from build123d import *

# Parameters (mm, degrees)
SKETCH1_R           = 2.5
BOSS_EXTRUDE1_DEPTH = 4
FILLET1_R           = 10.16


with BuildPart() as part:
    # Sketch1 → Boss-Extrude1 (new body)
    with BuildSketch(Plane(origin=(0, 25.4, 0), x_dir=(1, 0, 0), z_dir=(0, 1, 0))):
        Polygon((-190.5, -241.3), (-190.5, -279.4), (-190.5, -304.8), (-63.5, -304.8), (-63.5, -279.4), (-101.6, -279.4), (-101.6, -241.3), (-127, -241.3), (-127, -279.4), (-165.1, -279.4), (-165.1, -241.3), align=None)
        with Locations((-114.3, -292.1)):
            Circle(SKETCH1_R, mode=Mode.SUBTRACT)
        with Locations((-177.8, -292.1)):
            Circle(SKETCH1_R, mode=Mode.SUBTRACT)
        with Locations((-158.75, -292.1)):
            Circle(SKETCH1_R, mode=Mode.SUBTRACT)
        with Locations((-95.25, -292.1)):
            Circle(SKETCH1_R, mode=Mode.SUBTRACT)
        with Locations((-139.7, -292.1)):
            Circle(SKETCH1_R, mode=Mode.SUBTRACT)
        with Locations((-76.2, -292.1)):
            Circle(SKETCH1_R, mode=Mode.SUBTRACT)
        with Locations((-114.3, -273.05)):
            Circle(SKETCH1_R, mode=Mode.SUBTRACT)
        with Locations((-177.8, -273.05)):
            Circle(SKETCH1_R, mode=Mode.SUBTRACT)
        with Locations((-114.3, -254)):
            Circle(SKETCH1_R, mode=Mode.SUBTRACT)
        with Locations((-177.8, -254)):
            Circle(SKETCH1_R, mode=Mode.SUBTRACT)
    extrude(amount=BOSS_EXTRUDE1_DEPTH)

    # Fillet1
    fillet1_edges = [part.edges().sort_by_distance(p)[0] for p in [
        (-190.5, 27.4, 304.8),
        (-190.5, 27.4, 241.3),
        (-165.1, 27.4, 241.3),
        (-165.1, 27.4, 279.4),
        (-127, 27.4, 279.4),
        (-127, 27.4, 241.3),
        (-101.6, 27.4, 241.3),
        (-101.6, 27.4, 279.4),
        (-63.5, 27.4, 279.4),
        (-63.5, 27.4, 304.8),
    ]]
    fillet(fillet1_edges, radius=FILLET1_R)


solid = part.part
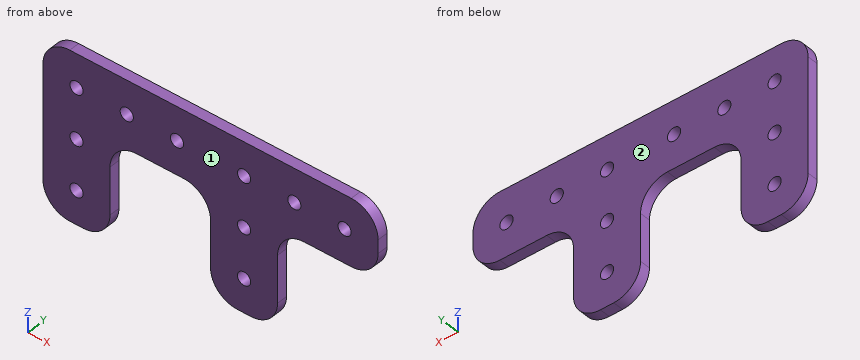
Build history of the part. All positions in model axes, mm. Face numbers are marked on the shaded views. Round coordinates to 2 decimals unless told otherwise and drop trailing zeros. Write each loop counter-clockwise with the first axis right and the second up, starting at its lowest first coordinate (ties: lowest second). Pieces come first, ordered by that corner, then holes. Notation, with made-up numbers: M 4,-0.75 L 59,-0.75 A10 ccw 59,4.25 Z; hole C 4,28 d11. An arc over 180 degrees is marked long. Use CSV: the item, a comma, the result in double quotes.
1. Saw through at C-C (x = -177.8). Give the cut face in (y, z), plus the area to 3 significant figures.
Reply:
outline,"M 25.4,241.3 L 29.4,241.3 L 29.4,251.5 L 25.4,251.5 Z; M 25.4,256.5 L 29.4,256.5 L 29.4,270.55 L 25.4,270.55 Z; M 25.4,275.55 L 29.4,275.55 L 29.4,289.6 L 25.4,289.6 Z; M 25.4,294.6 L 29.4,294.6 L 29.4,304.8 L 25.4,304.8 Z"
area,"194 mm²"
2. Saw through at A-A (z = 292.1). Give the cut face in (x, y).
Reply:
outline,"M -190.5,25.4 L -180.3,25.4 L -180.3,29.4 L -190.5,29.4 Z; M -175.3,25.4 L -161.25,25.4 L -161.25,29.4 L -175.3,29.4 Z; M -156.25,25.4 L -142.2,25.4 L -142.2,29.4 L -156.25,29.4 Z; M -137.2,25.4 L -116.8,25.4 L -116.8,29.4 L -137.2,29.4 Z; M -111.8,25.4 L -97.75,25.4 L -97.75,29.4 L -111.8,29.4 Z; M -92.75,25.4 L -78.7,25.4 L -78.7,29.4 L -92.75,29.4 Z; M -73.7,25.4 L -63.5,25.4 L -63.5,29.4 L -73.7,29.4 Z"
3. Wall check: probe 1 along X at (y, z) = (27.55, 254); probe 2 along Z at (x, y) = (-177.8, 28.1); probe 3 along X at (y, z) = (28.55, 258). Give the ranges that are in metal, low to high. Write a range as from..to.
Reply:
probe 1,"x = -190.5..-180.3, -175.3..-165.1, -127..-116.8, -111.8..-101.6"
probe 2,"z = 241.3..251.5, 256.5..270.55, 275.55..289.6, 294.6..304.8"
probe 3,"x = -190.5..-165.1, -127..-101.6"
4. Saw through at D-D (z = 265). Give the cut face in (x, y).
Reply:
outline,"M -190.5,25.4 L -165.1,25.4 L -165.1,29.4 L -190.5,29.4 Z; M -127,25.4 L -101.6,25.4 L -101.6,29.4 L -127,29.4 Z"
5. Two-plate mould, pull along Y, no slides. Class the marked faces 1 and 2: +Y half, -Y half, draft (parallel to the pull), parting line (faces both ways), or undercut.
Reply:
face 1,"-Y half"
face 2,"+Y half"
6. Flat gauge pins, fed straight in: pin 1 (4.5 mm diameter, centred on x = -114.3, z = 254, fed in from +Y); pin 2 (1.2 mm diameter, centred on y = 28, z = 261.5, fed in from +X); pin 3 (2 mm diameter, centred on x = -146.5, y = 28.5, fed in from -Z). Where does each tip first touch, or does it go through?
Reply:
pin 1,"passes through"
pin 2,"stops at x = -101.6"
pin 3,"stops at z = 279.4"
7. Saw through at B-B (x = -139.7). Give the cut face in (y, z), plus the area to 3 significant figures.
Reply:
outline,"M 25.4,279.4 L 29.4,279.4 L 29.4,289.6 L 25.4,289.6 Z; M 25.4,294.6 L 29.4,294.6 L 29.4,304.8 L 25.4,304.8 Z"
area,"81.6 mm²"
